Here's how the part is built. I have some questions about the finished solid (model axes, mm). Face numbers are marked on the shaded views. Coordinates: 2 decimals unless noted, no trailing zeros. Write each loop counter-clockwise with the first axis right and the second up, starting at its lowest first coordinate (ties: lowest second). Pieces come first, ordered by that corner, then holes. Notation, with made-up numbers: (-35.5, 34) - (4.5, 34) arc R8 ccw to (4.5, 47) - close; hole circle Ø10 at (-31, 81.5). An arc over 180 degrees is marked (long way). Answer in a Markdown table with one row per item. Add a question column.
Item 1: Imagine slicing it at A-A (z = 3). Please give me the cut outline in (x, y), plus the area to 3 significant figures.
Item 2: Imagine slicing it at D-D (z = -15.75). Please give me the cut outline in (x, y), plus the area to 3 significant figures.
Item 3: Imagine slicing it at B-B (y = -490). Please give me the cut outline in (x, z).
Item 4: If I drill on probe 1 along Z at (x, y) = (365.5, -489.5); probe 2 along Z at (x, y) = (363, -490.5); probe 3 along Y at (x, z) = (369.25, 3.25), over which ranges is the centre line in solid material (lowest first)? Write a range as from..to.
Item 5: We'd pull the mould along Y, two halves only. Please class the marked faces 1, 2, 3 and 4: +Y half, -Y half, draft (parallel to the pull), parting line (faces both ways), or undercut.
Item 6: Imagine slicing it at C-C (x = 366). Please give me the cut outline in (y, z).
Item 7: I'm going to push flat-ended pins straight in: pin 1 (1.5 mm diameter, centred on x = 369.5, y = -492.5, fed in from -Z); pin 2 (3 mm diameter, centred on y = -487.5, z = -15.5, fed in from -X); pin 3 (1 mm diameter, centred on x = 369, z = -13, fed in from -Y). Where does each tip first touch, or does it pass through?
from build123d import *

# Parameters (mm, degrees)
SKETCH1_R           = 5
BOSS_EXTRUDE1_DEPTH = 5
SKETCH2_R           = 2.5
BOSS_EXTRUDE2_DEPTH = 20
CUT_EXTRUDE1_DEPTH  = 4


with BuildPart() as part:
    # Sketch1 → Boss-Extrude1 (new body)
    with BuildSketch(Plane.XY):
        with Locations((367.033440134, -490)):
            Circle(SKETCH1_R)
    extrude(amount=BOSS_EXTRUDE1_DEPTH)

    # Sketch2 → Boss-Extrude2 (add)
    with BuildSketch(Plane(origin=(0, 0, 0), x_dir=(-1, 0, 0), z_dir=(0, 0, -1))):
        with Locations((-367.033440134, -490)):
            Circle(SKETCH2_R)
    extrude(amount=BOSS_EXTRUDE2_DEPTH)

    # Sketch3 → Cut-Extrude1 (cut)
    with BuildSketch(Plane.XY.offset(5)):
        Polygon((367.033440134, -493.218193517), (369.820477474, -491.609096758), (369.820477474, -488.390903242), (367.033440134, -486.781806483), (364.246402794, -488.390903242), (364.246402794, -491.609096758), align=None)
    extrude(amount=-CUT_EXTRUDE1_DEPTH, mode=Mode.SUBTRACT)


solid = part.part
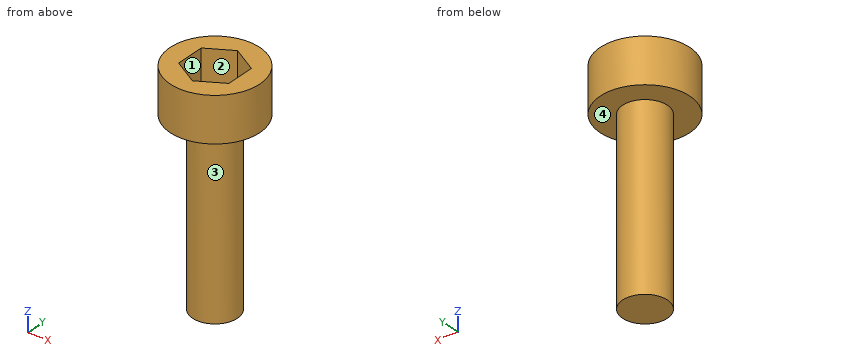
Here are the results:
| question | item | result |
|---|---|---|
| 1 | outline | circle Ø10 at (367.03, -490); hole (364.25, -491.61) - (367.03, -493.22) - (369.82, -491.61) - (369.82, -488.39) - (367.03, -486.78) - (364.25, -488.39) - close |
| 1 | area | 51.6 mm2 |
| 2 | outline | circle Ø5 at (367.03, -490) |
| 2 | area | 19.6 mm2 |
| 3 | outline | (362.03, 0) - (364.53, 0) - (364.53, -20) - (369.53, -20) - (369.53, 0) - (372.03, 0) - (372.03, 5) - (369.82, 5) - (369.82, 1) - (364.25, 1) - (364.25, 5) - (362.03, 5) - close |
| 4 | probe 1 | z = -20..1 |
| 4 | probe 2 | z = 0..5 |
| 4 | probe 3 | y = -494.48..-491.94, -488.06..-485.52 |
| 5 | face 1 | undercut |
| 5 | face 2 | undercut |
| 5 | face 3 | parting line |
| 5 | face 4 | draft |
| 6 | outline | (-494.89, 0) - (-492.28, 0) - (-492.28, -20) - (-487.72, -20) - (-487.72, 0) - (-485.11, 0) - (-485.11, 5) - (-487.38, 5) - (-487.38, 1) - (-492.62, 1) - (-492.62, 5) - (-494.89, 5) - close |
| 7 | pin 1 | stops at z = 0 |
| 7 | pin 2 | stops at x = 364.74 |
| 7 | pin 3 | stops at y = -492.02 |
